Here's how the part is built. I have some questions about the finished solid (model axes, mm). Give positions to 0.01 mm unless a question says otherwise; leave off trailing zeros. Loops run counter-clockwise (first coordinate to the right, second up) from the corner with the lowest first, then second, coordinate; pieces in that order, holes last. Notation, with made-up numbers: (-22.75, 57.25) - (-9.75, 57.25) arc R25 cw to (-9.75, 82.25) - close; hole circle Ø1 at (13.5, -8.75). An arc over 180 degrees is marked (long way). Use a Markdown table: item, result.
Autodesk Inventor part; units mm, degrees
ref_plane "YZ Plane" through (0, 0, 0) normal (1, 0, 0) x (0, 1, 0)
ref_plane "XZ Plane" through (0, 0, 0) normal (0, 1, 0) x (-1, 0, 0)
ref_plane "XY Plane" through (0, 0, 0) normal (0, 0, 1) x (1, 0, 0)
sketch "Sketch2" plane through (0, 0, 0) normal (0, 1, 0) x (-1, 0, 0)
  line L0 (90, -53) -> (84, -53)
  line L1 (84, -53) -> (84, -43)
  line L2 (84, -43) -> (90, -43)
  line L3 (-90, -53) -> (-84, -53)
  line L4 (-84, -53) -> (-84, -43)
  line L5 (-84, -43) -> (-90, -43)
  line L6 (70, -18) -> (60, -18)
  line L7 (60, -18) -> (60, -15)
  line L8 (60, -15) -> (70, -15)
  line L9 (70, -15) -> (70, -18)
  line L10 (-70, -18) -> (-60, -18)
  line L11 (-60, -18) -> (-60, -15)
  line L12 (-60, -15) -> (-70, -15)
  line L13 (-70, -15) -> (-70, -18)
  circle A0 centre (0, 0) radius 41.275
  line L14 (46.5, -15) -> (43.5, -15)
  line L15 (43.5, -15) -> (43.5, -5)
  line L16 (43.5, -5) -> (46.5, -5)
  line L17 (46.5, -5) -> (46.5, -15)
  line L18 (-46.5, -15) -> (-43.5, -15)
  line L19 (-43.5, -15) -> (-43.5, -5)
  line L20 (-43.5, -5) -> (-46.5, -5)
  line L21 (-46.5, -5) -> (-46.5, -15)
  line L22 (43.5, 57) -> (43.5, 47)
  line L23 (43.5, 47) -> (46.5, 47)
  line L24 (46.5, 47) -> (46.5, 57)
  line L25 (-46.5, 47) -> (-43.5, 47)
  line L26 (-43.5, 47) -> (-43.5, 57)
  line L27 (-46.5, 57) -> (-46.5, 47)
  line L28 (-85, 85) -> (85, 85)
  arc A1 (-85, 85) -> (-90, 80) centre (-85, 80) ccw
  arc A2 (90, 80) -> (85, 85) centre (85, 80) ccw
  line L29 (46.5, 57) -> (43.5, 57)
  line L30 (-43.5, 57) -> (-46.5, 57)
  line L31 (30, 57) -> (20, 57)
  line L32 (20, 57) -> (20, 60)
  line L33 (20, 60) -> (30, 60)
  line L34 (30, 60) -> (30, 57)
  line L35 (-20, 57) -> (-30, 57)
  line L36 (-30, 57) -> (-30, 60)
  line L37 (-30, 60) -> (-20, 60)
  line L38 (-20, 60) -> (-20, 57)
  line L39 (4.5, 70) -> (-4.5, 70)
  line L40 (-4.5, 70) -> (-4.5, 80)
  line L41 (-4.5, 80) -> (4.5, 80)
  line L42 (4.5, 80) -> (4.5, 70)
  line L43 (4.5, 45) -> (-4.5, 45)
  line L44 (-4.5, 45) -> (-4.5, 55)
  line L45 (-4.5, 55) -> (4.5, 55)
  line L46 (4.5, 55) -> (4.5, 45)
  line L47 (-90, -43) -> (-90, 80)
  line L48 (90, 80) -> (90, -43)
  line L49 (90, -53) -> (90, -65)
  line L50 (-90, -53) -> (-90, -65)
  line L51 (90, -65) -> (-90, -65)
  point P0 (90, 85)
  dimension "d21" = 6
  dimension "d22" = 10
  dimension "d25" = 6
  dimension "d26" = 10
  dimension "d31" = 3
  dimension "d32" = 10
  dimension "d35" = 3
  dimension "d36" = 10
  dimension "d39" = 25
  dimension "d40" = 25
  dimension "d43" = 82.55
  dimension "d52" = 3
  dimension "d53" = 10
  dimension "d54" = 10
  dimension "d55" = 3
  dimension "d58" = 10
  dimension "d59" = 3
  dimension "d62" = 3
  dimension "d65" = 180
  dimension "d66" = 150
  dimension "d90" = 90
  dimension "d91" = 90
  dimension "d103" = 10
  dimension "d104" = 10
  dimension "d108" = 3
  dimension "d109" = 10
  dimension "d110" = 20
  dimension "d111" = 3
  dimension "d112" = 10
  dimension "d113" = 20
  dimension "d114" = 5
  dimension "d115" = 10
  dimension "d116" = 9
  dimension "d117" = 4.5
  dimension "d118" = 10
  dimension "d119" = 9
  dimension "d120" = 15
  dimension "d121" = 4.5
  dimension "d127" = 180
  dimension "d128" = 150
  dimension "d130" = 85.5
  dimension "d131" = 43.5
  dimension "d132" = 43.5
  dimension "d133" = 60
  dimension "d134" = 60
  dimension "d135" = 43.5
  dimension "d136" = 43.5
  dimension "d137" = 90
  dimension "d138" = 28
  dimension "d140" = 47
  dimension "d141" = 47
extrude "Extrusion6" add sketch "Sketch2" along normal blind 3
properties part number "OpenROV 2_3 Dev Top"
(1) Suppose I cut it at A-A on z = 0. Write out the boundary of the cut face in (x, y) (3 decimals), plus the area to 3 significant figures.
A:
| item | result |
|---|---|
| outline | (-90, 0) - (-41.275, 0) - (-41.275, 3) - (-90, 3) - close; (41.275, 0) - (90, 0) - (90, 3) - (41.275, 3) - close |
| area | 292 mm2 |
(2) If I drill on line 1 (Z direction, x = 0, y = 1.05) (3 decimals); line 2 (X direction, y = 2.25, z = 54.5); line 3 (X direction, y = 2.2, z = 71), over which ranges is the centre line in solid material (lowest first)?
A:
| item | result |
|---|---|
| line 1 | -65 to -41.275, 41.275 to 45, 55 to 70, 80 to 85 |
| line 2 | -90 to -46.5, -43.5 to -4.5, 4.5 to 43.5, 46.5 to 90 |
| line 3 | -90 to -4.5, 4.5 to 90 |
(3) Will this pin go through, and if not, where does the flat tip stop? pin 1 (0.9 mm diameter, centred on x = -86, y = 1.5, fed in from +Z).
A:
| item | result |
|---|---|
| pin 1 | z = 84.97 |
(4) Suppose I cut it at B-B on x = 0. Write out the boundary of the cut face in (y, z) (3 decimals).
A:
| item | result |
|---|---|
| outline | (0, -65) - (3, -65) - (3, -41.275) - (0, -41.275) - close; (0, 41.275) - (3, 41.275) - (3, 45) - (0, 45) - close; (0, 55) - (3, 55) - (3, 70) - (0, 70) - close; (0, 80) - (3, 80) - (3, 85) - (0, 85) - close |
(5) Suppose I cut it at D-D on z = 33.5. Write out the boundary of the cut face in (x, y), plus the area to 3 significant figures.
A:
| item | result |
|---|---|
| outline | (-90, 0) - (-24.11, 0) - (-24.11, 3) - (-90, 3) - close; (24.11, 0) - (90, 0) - (90, 3) - (24.11, 3) - close |
| area | 395 mm2 |
(6) We'd pull the mould along X, two halves only. Please class faces 1 (the face through (-88, 1, 84)), 2 (the face through (8.948, 1.479, 40.293)), 3 (the face through (89, 1, 83)): pulls with the +X half, pulls with the -X half, needs draft (parallel to the pull), parting line crosses it, or undercut.
A:
| item | result |
|---|---|
| face 1 | pulls with the -X half |
| face 2 | undercut |
| face 3 | pulls with the +X half |
(7) Suppose I cut it at C-C on y = 1.85. Count the separate pieces of the cut face and the enclosed holes in it, plus the area to 3 significant figures.
A:
| item | result |
|---|---|
| separate pieces | 1 |
| enclosed holes | 11 |
| area | 21,100 mm2 |
